Source: CAD feature listing. Evaluate the final solid. Frame: model axes, mm. A direction names the side the tool comes from. Round coordinates to 2 decimals unless told otherwise and drop trailing zeros. Order: outer loops, then holes, each group sorted by start corner. A loop starts at its lowest first (then second) coordinate and runs counter-clockwise, first axis right, second up. Notation, with made-up numbers: (15, -5.5) - (73, -5.5) arc R10 ccw to (73, 13.5) - close; hole circle Ø8 at (-13, 3.25). An arc over 180 degrees is marked (long way). Put each result on its own line as item: value. Start each with the question number.
1) Mould query, pull axis Y, two halves, no side actions, for faces 6 (the face through (2.655, -17.344, 1.565)), 7 (the face through (4.48, 15.09, 1.57)), 8 (the face through (-15.104, -4.477, 1.565)). Classes: +Y half, -Y half, draft (parallel to the pull), parting line (faces both ways), or undercut.
2) Contact query for flat-ended pins moving along their axis: P1, Ø4, axis at x = -3, y = 7.5, coming from the +Z side (3 decimals); P2, Ø2.5, axis at x = -6.93, y = -4, coming from the -Z side; P3, Ø1, axis at x = -10.5, z = 3, coming from the +Y side; P4, Ø5.5, axis at x = 6.93, y = -4, coming from the +Z side. Output: stop coordinate, or through.
3) Line query: probe 1 along Y at (x, z) = (-7, 1.3); probe 2 along Y at (x, z) = (1, 1.2); probe 3 along X at (y, z) = (-4, 0.9). Output: solid intervals per line, ascending. Write a range as [from, to].
4) Access query for faces 1 (the face through (9.09, -15.007, 1.565)), 2 (the face through (15.104, 4.477, 1.565)), 3 (the face through (-10.323, -10.293, 1.565)), 4 (the face through (-12.226, 9.913, 1.565)), 5 (the face through (-9.913, -12.226, 1.565)). Directions: +Z, -Z, +X, -X, +Y, -Y. A direction counts if a zero-diameter tool reaches every point of the face in a straight line with its end or side. Return the directions, or none.
5) Section B-B on z = 1.1. State how many separate pieces and enclosed holes the cut face has, then the cut area to 3 significant figures.
6) Section A-A on y = 4. Output: boundary loops of the cut face in (x, z) (3 decimals), then the cut area to 3 significant figures.
```python
from build123d import *

# Parameters (mm, degrees)
SKETCH3_R                    = 18.654838605
BOSS_EXTRUDE1_DEPTH          = 3.175
CUT_EXTRUDE1_START           = -1
CUT_EXTRUDE1_DEPTH           = 5.175
CIRPATTERN1_COUNT            = 16
CSK_FOR_M3_SFHCS1_AT_2_COUNT = 2
CSK_FOR_M3_SFHCS1_AT_2_PITCH = 8
CSK_FOR_M3_SFHCS1_AT_3_COUNT = 2
CSK_FOR_M3_SFHCS1_AT_3_PITCH = 13.856406461
CSK_FOR_M3_SFHCS1_AT_4_COUNT = 2
CSK_FOR_M3_SFHCS1_AT_4_PITCH = 16
CSK_FOR_M3_SFHCS1_AT_5_COUNT = 2
CSK_FOR_M3_SFHCS1_AT_5_PITCH = 13.856406461
CSK_FOR_M3_SFHCS1_AT_6_COUNT = 2
CSK_FOR_M3_SFHCS1_AT_6_PITCH = 8


with BuildPart() as part:
    # Sketch3 → Boss-Extrude1 (new body)
    with BuildSketch(Plane.XY):
        Circle(SKETCH3_R)
    extrude(amount=BOSS_EXTRUDE1_DEPTH)

    # Sketch2 → Cut-Extrude1 (cut)
    with BuildSketch(Plane.XY.offset(CUT_EXTRUDE1_START)):
        with BuildLine():
            Line((101.443267524, 18.095471295), (4.533974194, 18.095471295))
            ThreePointArc((4.533974194, 18.095471295), (3.056004647, 17.659429879), (2.051408678, 16.490963774))
            Line((2.051408678, 16.490963774), (1.895951627, 16.145861918))
            ThreePointArc((1.895951627, 16.145861918), (1.639424454, 15.660854777), (1.323740827, 15.212098758))
            ThreePointArc((1.323740827, 15.212098758), (0, 14.577158093), (-1.323740827, 15.212098758))
            ThreePointArc((-1.323740827, 15.212098758), (-1.639424454, 15.660854777), (-1.895951627, 16.145861918))
            Line((-1.895951627, 16.145861918), (-2.051408678, 16.490963774))
            ThreePointArc((-2.051408678, 16.490963774), (-3.056004647, 17.659429879), (-4.533974194, 18.095471295))
            Line((-4.533974194, 18.095471295), (-101.443267524, 18.095471295))
            Line((-101.443267524, 18.095471295), (-101.443267524, 211.914057954))
            Line((-101.443267524, 211.914057954), (101.443267524, 211.914057954))
            Line((101.443267524, 211.914057954), (101.443267524, 18.095471295))
        make_face()
    cut_extrude1 = extrude(amount=CUT_EXTRUDE1_DEPTH, mode=Mode.SUBTRACT)

    # CirPattern1: Cut-Extrude1 ×16 about axis
    cirpattern1_axis = Axis((0, 0, -80.9), (0, 0, 1))
    for i in range(1, CIRPATTERN1_COUNT):
        add(cut_extrude1.rotate(cirpattern1_axis, i * 360 / CIRPATTERN1_COUNT), mode=Mode.SUBTRACT)

    # Sketch5 → CSK for M3 SFHCS1 (revolve, cut)
    with BuildSketch(Plane(origin=(0, 8, 3.175), x_dir=(0, -1, 0), z_dir=(1, 0, 0))):
        Polygon((0, 0), (0, 3.175), (1.7, 3.175), (1.7, 1.66), (3.36, 0), align=None)
    csk_for_m3_sfhcs1 = revolve(axis=Axis((0, 8, 9.525), (0, 0, -1)), mode=Mode.SUBTRACT)

    # CSK for M3 SFHCS1 at 2: CSK for M3 SFHCS1 ×2
    with Locations(*[Vector(0.866025404, -0.5, 0) * (i * CSK_FOR_M3_SFHCS1_AT_2_PITCH) for i in range(1, CSK_FOR_M3_SFHCS1_AT_2_COUNT)]):
        add(csk_for_m3_sfhcs1, mode=Mode.SUBTRACT)

    # CSK for M3 SFHCS1 at 3: CSK for M3 SFHCS1 ×2
    with Locations(*[Vector(0.5, -0.866025404, 0) * (i * CSK_FOR_M3_SFHCS1_AT_3_PITCH) for i in range(1, CSK_FOR_M3_SFHCS1_AT_3_COUNT)]):
        add(csk_for_m3_sfhcs1, mode=Mode.SUBTRACT)

    # CSK for M3 SFHCS1 at 4: CSK for M3 SFHCS1 ×2
    with Locations(*[(0, -i * CSK_FOR_M3_SFHCS1_AT_4_PITCH, 0) for i in range(1, CSK_FOR_M3_SFHCS1_AT_4_COUNT)]):
        add(csk_for_m3_sfhcs1, mode=Mode.SUBTRACT)

    # CSK for M3 SFHCS1 at 5: CSK for M3 SFHCS1 ×2
    with Locations(*[Vector(-0.5, -0.866025404, 0) * (i * CSK_FOR_M3_SFHCS1_AT_5_PITCH) for i in range(1, CSK_FOR_M3_SFHCS1_AT_5_COUNT)]):
        add(csk_for_m3_sfhcs1, mode=Mode.SUBTRACT)

    # CSK for M3 SFHCS1 at 6: CSK for M3 SFHCS1 ×2
    with Locations(*[Vector(-0.866025404, -0.5, 0) * (i * CSK_FOR_M3_SFHCS1_AT_6_PITCH) for i in range(1, CSK_FOR_M3_SFHCS1_AT_6_COUNT)]):
        add(csk_for_m3_sfhcs1, mode=Mode.SUBTRACT)


solid = part.part
```
Answer sheet:
1. face 6: -Y half
1. face 7: +Y half
1. face 8: undercut
2. P1: z = 3.175
2. P2: through
2. P3: y = 15.19
2. P4: z = 2.57
3. probe 1: [-13.52, -5.7], [-2.3, 2.3], [5.7, 13.52]
3. probe 2: [-14.9, -9.37], [-6.63, 6.63], [9.37, 14.9]
3. probe 3: [-17.39, -8.63], [-5.23, 5.23], [8.63, 17.39]
4. face 1: +Z, -Z, -Y
4. face 2: +Z, -Z, +X
4. face 3: +Z, -Z
4. face 4: +Z, -Z, +Y
4. face 5: +Z, -Z, -X
5. separate pieces: 1
5. enclosed holes: 6
5. area: 759 mm^2
6. outline: (-17.385, 0) - (-8.628, 0) - (-8.628, 1.515) - (-10.288, 3.175) - (-17.385, 3.175) - close; (-5.228, 0) - (5.228, 0) - (5.228, 1.515) - (3.568, 3.175) - (-3.568, 3.175) - (-5.228, 1.515) - close; (8.628, 0) - (17.385, 0) - (17.385, 3.175) - (10.288, 3.175) - (8.628, 1.515) - close
6. area: 83.3 mm^2
